Input: dimensioned drawing with shaded views. Units: mm. Origin: part minimum x, y, z. A direction names the side the tool comes from. Coordinates: 2 decimals unless noted, no trailing zeros. Loops run counter-clockwise (first coordinate to the right, second up) from the corner with the lowest first, then second, coordinate; pieces in that order, holes last.
Item 1: Pull-direction query (X, two-part tool) for the marked faces 4, 5 and 6; classes: released by +X, released by -X, zero draft, split by the parting line, or undercut.
Item 2: Section C-C on x = 17.75. Return loops of the section in (y, z).
Item 3: Section B-B on z = 5. Return loops of the section in (x, y), and give its area (3 significant figures).
Item 4: Ray query, line 1 along X through (y, z) = (0.9, 5); line 2 along X through (y, z) = (2.95, 5); line 3 along X through (y, z) = (19.25, 21.25). Return the intervals inside material, ascending.
Item 5: Contact query for flat-ended pins moving along their axis: P1, Ø9, axis at x = 3.5, z = 5.5, coming from the +Y side; P2, Ø6.5, axis at y = 20, z = 18.5, coming from the -X side; P3, Ø12, axis at y = 12.5, z = 20, coming from the +X side. Output: stop coordinate, or through.
Item 6: Section A-A on y = 13. Return loops of the section in (x, z), and give its area (3 significant figures).
Item 7: Section D-D on y = 21. Return loops of the section in (x, z), and give its area (3 significant figures).
Item 8: Reachability of the marked faces 1, 2 and 3 from +Z, -Z, +X, -X, +Y, -Y: full face, straight path, thin tool, end or side. Return the list, or none.
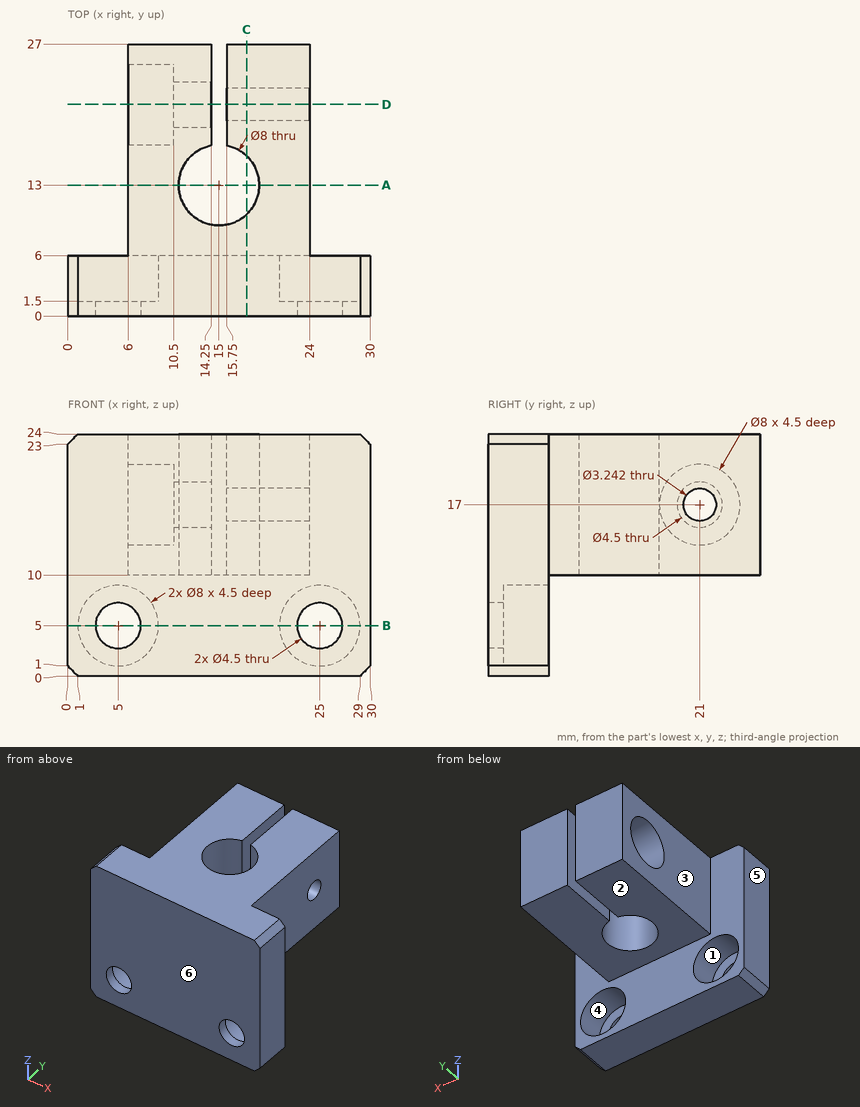
Results found:
1. face 4: undercut
1. face 5: released by -X
1. face 6: zero draft
2. outline: (0, 0) - (6, 0) - (6, 10) - (10.1, 10) - (10.1, 24) - (0, 24) - close; (15.9, 10) - (27, 10) - (27, 24) - (15.9, 24) - close; hole circle Ø3.24 at (21, 17)
3. outline: (0, 0) - (2.75, 0) - (2.75, 1.5) - (1, 1.5) - (1, 6) - (0, 6) - close; (7.25, 0) - (22.75, 0) - (22.75, 1.5) - (21, 1.5) - (21, 6) - (9, 6) - (9, 1.5) - (7.25, 1.5) - close; (27.25, 0) - (30, 0) - (30, 6) - (29, 6) - (29, 1.5) - (27.25, 1.5) - close
3. area: 94.5 mm2
4. line 1: x = 0 to 2.75, 7.25 to 22.75, 27.25 to 30
4. line 2: x = 0 to 1, 9 to 21, 29 to 30
4. line 3: x = 6 to 14.25, 15.75 to 24
5. P1: stops at y = 6
5. P2: stops at x = 6
5. P3: stops at x = 24
6. outline: (6, 10) - (11, 10) - (11, 24) - (6, 24) - close; (19, 10) - (24, 10) - (24, 24) - (19, 24) - close
6. area: 140 mm2
7. outline: (6, 10) - (14.25, 10) - (14.25, 14.75) - (10.5, 14.75) - (10.5, 13) - (6, 13) - close; (6, 21) - (10.5, 21) - (10.5, 19.25) - (14.25, 19.25) - (14.25, 24) - (6, 24) - close; (15.75, 10) - (24, 10) - (24, 15.38) - (15.75, 15.38) - close; (15.75, 18.62) - (24, 18.62) - (24, 24) - (15.75, 24) - close
7. area: 151 mm2
8. face 1: +Y
8. face 2: -Z, +X, -X, +Y
8. face 3: +Z, -Z, -X, +Y
